Can you work these out from the drawing? Everything is in mm from the part's minimum corner. A direction names the side the tool comes from. Round coordinates to 2 decimals unless told otherwise and drop trailing zeros. Loops run counter-clockwise (first coordinate to the right, second up) from the corner with the lowest first, then second, coordinate; pieces in that order, holes last. Notation, with made-up numbers: M -1,20.25 L 53,20.25 A12 cw 53,36.25 Z; hole C 55,29 d9. An arc over 180 degrees is marked long. Use a Markdown table: item, result.
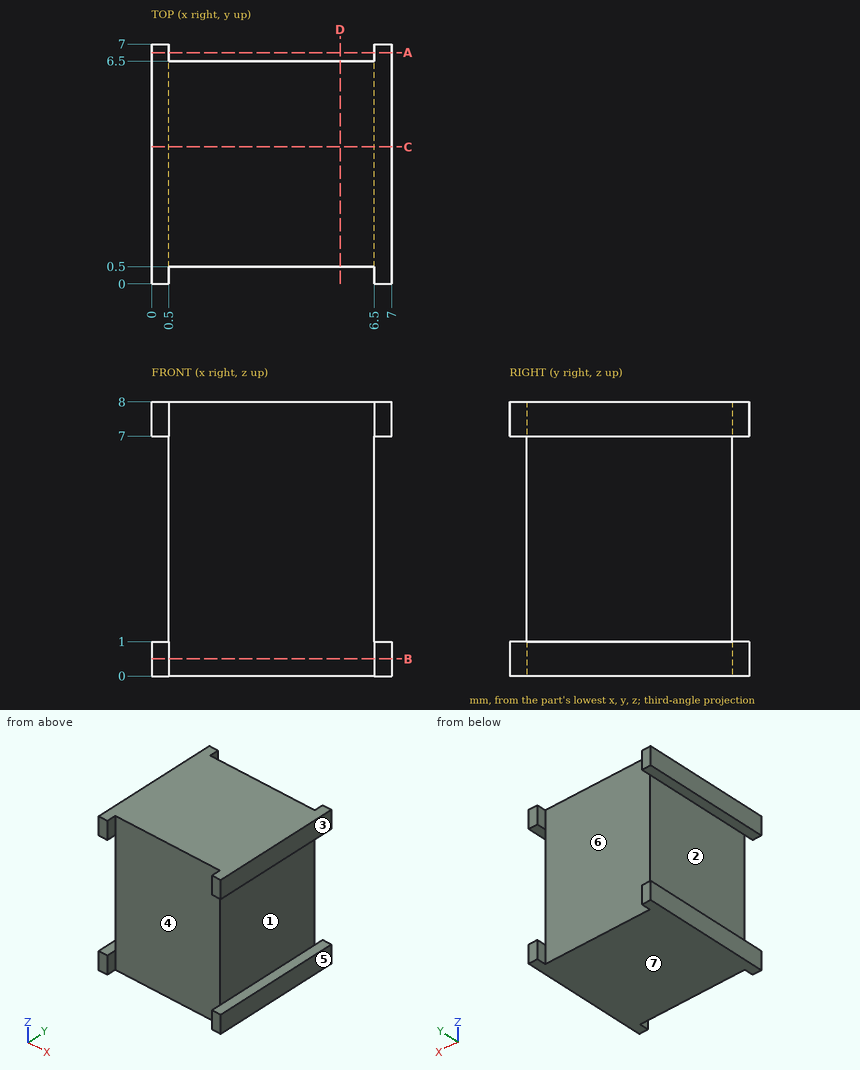
1. Which directions (+Z, -Z, +X, -X, +Y, -Y) give clear straight access to the entire face, cutting with the end or side of a thin tool? Please do the marked faces 1, 2 and 3.
Answer sheet:
| item | result |
|---|---|
| face 1 | +X, +Y, -Y |
| face 2 | -X, +Y, -Y |
| face 3 | +Z, -Z, +X, +Y, -Y |
2. We'd pull the mould along X, two halves only. Please class the marked faces 4, 5, 6 and 7: +X half, -X half, draft (parallel to the pull), parting line (faces both ways), or undercut.
Answer sheet:
| item | result |
|---|---|
| face 4 | undercut |
| face 5 | +X half |
| face 6 | undercut |
| face 7 | draft |
3. For pin 1 Ø1.5 at (x, z) = (4.5, 3) entering from -Y; pin 2 Ø3 at (y, z) = (1, 5) entering from -X; pin 3 Ø3 at (y, z) = (4.5, 4.5) entering from +X, each with a flat end and sliding along its axis, tell me the tip position at first contact or that it passes through.
Answer sheet:
| item | result |
|---|---|
| pin 1 | y = 0.5 |
| pin 2 | x = 0.5 |
| pin 3 | x = 6.5 |
4. Imagine slicing it at D-D, the plane x = 5.5. Write out the boundary of the cut face in (y, z).
Answer sheet:
| item | result |
|---|---|
| outline | M 0.5,0 L 6.5,0 L 6.5,8 L 0.5,8 Z |
5. Imagine slicing it at C-C, the plane y = 4. Write out the boundary of the cut face in (x, z), then the cut area to 3 significant figures.
Answer sheet:
| item | result |
|---|---|
| outline | M 0,0 L 7,0 L 7,1 L 6.5,1 L 6.5,7 L 7,7 L 7,8 L 0,8 L 0,7 L 0.5,7 L 0.5,1 L 0,1 Z |
| area | 50.0 mm2 |
6. Imagine slicing it at B-B, the plane z = 0.5. Write out the boundary of the cut face in (x, y).
Answer sheet:
| item | result |
|---|---|
| outline | M 0,0 L 0.5,0 L 0.5,0.5 L 6.5,0.5 L 6.5,0 L 7,0 L 7,7 L 6.5,7 L 6.5,6.5 L 0.5,6.5 L 0.5,7 L 0,7 Z |
7. I need wall thicknesses on probe 1 along X at (y, z) = (4.5, 4.5). Which ranges of the line are inside material? Lowest first, please. Write a range as from..to.
Answer sheet:
| item | result |
|---|---|
| probe 1 | 0.5..6.5 |
8. Imagine slicing it at A-A, the plane y = 6.75. Write out the boundary of the cut face in (x, z).
Answer sheet:
| item | result |
|---|---|
| outline | M 0,0 L 0.5,0 L 0.5,1 L 0,1 Z; M 0,7 L 0.5,7 L 0.5,8 L 0,8 Z; M 6.5,0 L 7,0 L 7,1 L 6.5,1 Z; M 6.5,7 L 7,7 L 7,8 L 6.5,8 Z |
